Autodesk Fusion 360 part; units mm, degrees
sketch "スケッチ1" plane through (0, 0, 0) normal (0, 0, 1) x (1, 0, 0)
  line L0 (-3.5, 163) -> (-86.5, 163)
  line L1 (-86.5, 163) -> (-86.5, -163)
  line L2 (-86.5, -163) -> (-3.5, -163)
  line L3 (86.5, -155) -> (86.5, 155)
  line L4 (82.2546, 155) -> (-86.5, -163) construction
  line L5 (-86.5, 163) -> (82.2546, -155) construction
  line L6 (-3.5, 163) -> (-3.5, 155)
  line L7 (-3.5, 155) -> (86.5, 155)
  line L8 (-3.5, -163) -> (-3.5, -155)
  line L9 (-3.5, -155) -> (86.5, -155)
  dimension "d2" = 326
extrude "押し出し1" add sketch "スケッチ1" along normal blind 9
chamfer "面取り1" distance 30 angle 45 2 edges at (-86.5, -163, 4.5) (-86.5, 163, 4.5)
sketch "スケッチ2" plane through (0, 0, 9) normal (0, 0, 1) x (-1, 0, 0)
  line L0 (56.5, -163) -> (86.5, -133)
  line L1 (86.5, -133) -> (86.5, 133)
  line L2 (86.5, 133) -> (56.5, 163)
  line L3 (56.5, 163) -> (3.5, 163)
  line L4 (3.5, 163) -> (3.5, 155)
  line L5 (3.5, 155) -> (-86.5, 155)
  line L6 (-86.5, 155) -> (-86.5, -155)
  line L7 (-86.5, -155) -> (3.5, -155)
  line L8 (3.5, -155) -> (3.5, -163)
  line L9 (3.5, -163) -> (56.5, -163)
  line L10 (-86.5, -155) -> (-46.5, -155) construction
  line L11 (-46.5, -155) -> (-46.5, -105) construction
  line L12 (-46.5, -105) -> (-86.5, -105) construction
  line L13 (-86.5, -105) -> (-86.5, -155) construction
  line L14 (-46.5, -105) -> (-46.5, -35) construction
  line L15 (-86.5, 0) -> (101.7247, 0)
  point P0 (-46.5, -105)
  point P1 (-46.5, -35)
  point P2 (-46.5, 105)
  point P3 (-46.5, 35)
  dimension "d10" = 40
  dimension "d11" = 50
  dimension "d12" = 70
hole "穴1" at (46.5, 105, 9) at (46.5, 35, 9) at (46.5, -35, 9) at (46.5, -105, 9) direction (0, 0, -1) diameter 22 end through all
Geometry: final body of the model. Coordinates: model frame, mm. A direction names the side the tool comes from. Give positions to 0.01 mm unless a question says otherwise; leave off trailing zeros. Write each loop counter-clockwise with the first axis right and the second up, starting at its lowest first coordinate (ties: lowest second). Pieces come first, ordered by that corner, then holes.
(1) First-contact query: P1, Ø2.5, axis at x = 47, z = 5, coming from the -Y side; P2, Ø4, axis at y = 158.5, z = 6.5, coming from the +X side; P3, Ø20, axis at x = 46.5, y = -105, coming from the +Z side; P4, Ø3, axis at x = 49.5, z = 5, coming from the +Y side. Flat tips, straight axial feed; report the tip coordinate or a pass-through.
(2) Cut plane A-A, the plane y = 35. Return loops of the section in (x, z).
(3) Access query for faces 4 (the flat face through (-3.5, -159, 4)), 5 (the flat face through (-3.5, 159, 4)), 6 (the cylindrical face through (46.02, 115.99, 4.44)). Directions: +Z, -Z, +X, -X, +Y, -Y. A direction counts if a zero-diameter tool reaches every point of the face in a straight line with its end or side. Return the directions, or none.
(4) Ray query, line 1 (Y direction, x = 46.5, z = 3); line 2 (X direction, y = -35, z = 2); line 3 (Y direction, x = 15.5, z = 2.5). Return the intervals inside material, ascending.
(5) Cut plane B-B, the plane x = 46.5. Return loops of the section in (y, z).
(6) Mould query, pull axis X, two halves, no side actions, for faces 1 (the cylindrical face through (39.07, -26.89, 4.44)), 2 (the flat face through (-71.7, -147.8, 4.4)), 3 (the flat face through (-1, 2, 9)). Classes: released by +X, released by -X, zero draft, split by the parting line, or undercut.
(7) Cut plane C-C, the plane z = 4.5. Return loops of the section in (x, y), then the cut area to 3 significant figures.
(8) Cut plane D-D, the plane x = 24. Return loops of the section in (y, z).
Values follow:
1. P1: stops at y = -155
1. P2: stops at x = -3.5
1. P3: passes through
1. P4: stops at y = 155
2. outline: (-86.5, 0) - (35.5, 0) - (35.5, 9) - (-86.5, 9) - close; (57.5, 0) - (86.5, 0) - (86.5, 9) - (57.5, 9) - close
3. face 4: +Z, -Z, +X, -Y
3. face 5: +Z, -Z, +X, +Y
3. face 6: +Z, -Z
4. line 1: y = -155 to -116, -94 to -46, -24 to 24, 46 to 94, 116 to 155
4. line 2: x = -86.5 to 35.5, 57.5 to 86.5
4. line 3: y = -155 to 155
5. outline: (-155, 0) - (-116, 0) - (-116, 9) - (-155, 9) - close; (-94, 0) - (-46, 0) - (-46, 9) - (-94, 9) - close; (-24, 0) - (24, 0) - (24, 9) - (-24, 9) - close; (46, 0) - (94, 0) - (94, 9) - (46, 9) - close; (116, 0) - (155, 0) - (155, 9) - (116, 9) - close
6. face 1: undercut
6. face 2: released by -X
6. face 3: zero draft
7. outline: (-86.5, -133) - (-56.5, -163) - (-3.5, -163) - (-3.5, -155) - (86.5, -155) - (86.5, 155) - (-3.5, 155) - (-3.5, 163) - (-56.5, 163) - (-86.5, 133) - close; hole circle Ø22 at (46.5, -105); hole circle Ø22 at (46.5, -35); hole circle Ø22 at (46.5, 35); hole circle Ø22 at (46.5, 105)
7. area: 52,500 mm2
8. outline: (-155, 0) - (155, 0) - (155, 9) - (-155, 9) - close
